Here's how the part is built. I have some questions about the finished solid (model axes, mm). A direction names the side the tool comes from. Round coordinates to 2 decimals unless told otherwise and drop trailing zeros. Loops run counter-clockwise (first coordinate to the right, second up) from the corner with the lowest first, then second, coordinate; pieces in that order, holes last. Notation, with made-up numbers: (-21.75, 40.25) -> (33.25, 40.25) arc R20 ccw to (33.25, 70.25) -> close; hole circle Ø7 at (15, 30.25). An arc over 180 degrees is marked (long way). Use one line per item in the form item = value. Start each with the question number.
Item 1: For faces 4 (the face through (-17, -1.6, -3.3)), 5 (the face through (-0.6, 1.2, 5.9)), 6 (the face through (0, -7.5, 0)), which set-ups out of +Z, -Z, +X, -X, +Y, -Y let a thin tool reach every point of the face, with its end or its side?
Item 2: Thinking about a two-plate mould opening in X: for faces 1 (the face through (-24.16, 6.99, 0.46)), 2 (the face through (-0.4, 0.84, 6.46)), 3 (the face through (0, 7.5, 0)), which applies, released by +X, released by -X, zero draft, split by the parting line, or undercut?
Item 3: If I drill on L1, parallel to X at y = -1.7, z = 1; L2, parallel to X at y = -3.75, z = -3; L3, parallel to Y at x = 20, z = 1.25, over which ranges is the centre line in solid material (lowest first)? Write a range as [from, to].
Item 4: If we section it at B-B (z = 2.75): Write out the boundary of the cut face in (x, y).
Item 5: If we section it at D-D (y = -1.7): State how many separate pieces and enclosed holes the cut face has, then the cut area to 3 significant figures.
Item 6: If we section it at A-A (x = -20): Write out the boundary of the cut face in (y, z), then the cut area to 3 significant figures.
Item 7: If we section it at C-C (x = 13.5): Write out the boundary of the cut face in (y, z).
Item 8: I'm going to push flat-ended pins straight in: pin 1 Ø2 at (x, z) = (-2, 6.5) entering from -Y; pin 2 Ø8 at (x, y) = (20, -1.7) entering from +Z; pin 3 Ø5.5 at (y, z) = (-2, 8) entering from +X. Where does each tip first touch, or does it pass through?
Autodesk Inventor part; units mm, degrees
ref_plane "YZ Plane" through (0, 0, 0) normal (1, 0, 0) x (0, 1, 0)
ref_plane "XZ Plane" through (0, 0, 0) normal (0, 1, 0) x (-1, 0, 0)
ref_plane "XY Plane" through (0, 0, 0) normal (0, 0, 1) x (1, 0, 0)
sketch "Sketch1" plane through (0, 0, 0) normal (0, 0, 1) x (1, 0, 0)
  line L0 (-24.65, 7.5) -> (24.65, 7.5)
  line L1 (24.65, 7.5) -> (24.65, -7.5)
  line L2 (24.65, -7.5) -> (-24.65, -7.5)
  line L3 (-24.65, -7.5) -> (-24.65, 7.5)
  circle A0 centre (-20, -1.7) radius 2
  circle A1 centre (20, -1.7) radius 2
  point P0 (0, 0)
  point P1 (-24.65, 0)
  point P2 (0, 7.5)
  dimension "d0" = 49.3
  dimension "d1" = 15
  dimension "d2" = 4
  dimension "d3" = 40
  dimension "d7" = 9.2
  dimension "d8" = 9.2
  dimension "d9" = 20
extrude "Extrusion1" add sketch "Sketch1" along normal mid plane 9.5
sketch "Sketch2" plane through (0, 0, 4.75) normal (0, 0, 1) x (1, 0, 0)
  line L0 (-6.65, 1.2) -> (5.65, 1.2)
  line L1 (5.65, 1.2) -> (5.65, -4.6)
  line L2 (5.65, -4.6) -> (-6.65, -4.6)
  line L3 (-6.65, -4.6) -> (-6.65, 1.2)
  line L4 (-24.65, 7.5) -> (24.65, 7.5)
  line L5 (24.65, -7.5) -> (24.65, 7.5)
  line L6 (-6.5, 1.2) -> (-6.5, -4.6)
  line L7 (-24.65, -7.5) -> (24.65, -7.5)
  line L8 (5.5, 1.2) -> (5.5, -4.6)
  point P0 (0, 0)
  dimension "d10" = 5.8
  dimension "d11" = 6.3
  dimension "d12" = 12.3
  dimension "d13" = 19
  dimension "d14" = 0.15
extrude "Extrusion3" add sketch "Sketch2" along normal blind 8 contours L0 L8 L2 L6
sketch "Sketch3" plane through (-6.5, 1.2, 4.75) normal (0, 1, 0) x (1, 0, 0)
  line L0 (0, -8) -> (12, -8)
  circle A0 centre (6, -8) radius 6.15
  point P0 (6.5, 4.75)
  dimension "d20" = 12.3
extrude "Extrusion4" cut sketch "Sketch3" against normal blind 8
chamfer "Chamfer1" distance 0.5 angle 45 4 edges at (-6.5, -4.6, 8.075) (-6.5, 1.2, 8.075) (5.5, 1.2, 8.075) (5.5, -4.6, 8.075)
chamfer "Chamfer2" distance 0.5 angle 45 2 edges at (-0.5, -4.6, 6.6) (-0.5, 1.2, 6.6)
fillet "Fillet1" radius 0.2 2 edges at (-6.5, -1.7, 11.4) (5.5, -1.7, 11.4)
chamfer "Chamfer3" distance 1 angle 45 8 edges at (24.65, 0, -4.75) (-24.65, 0, -4.75) (0, 7.5, -4.75) (24.65, 7.5, 0) (-24.65, 7.5, 0) (24.65, -7.5, 0) (0, -7.5, -4.75) (-24.65, -7.5, 0)
sketch "Sketch4" plane through (0, 0, -4.75) normal (0, 0, -1) x (-1, 0, 0)
  circle A0 centre (-20, -1.7) radius 2
  circle A1 centre (-20, -1.7) radius 3
  circle A2 centre (20, -1.7) radius 2
  circle A3 centre (20, -1.7) radius 3
  point P0 (0, 0)
  dimension "d33" = 6
  dimension "d34" = 6
extrude "Extrusion5" cut sketch "Sketch4" against normal blind 3 contours A0 | A1 | A2 | A3
fillet "Fillet2" radius 0.2 8 edges at (0, 7.5, 4.75) (0, -7.5, 4.75) (-24.65, 0, 4.75) (24.65, 0, 4.75) (24.15, 7, 4.75) (24.15, -7, 4.75) (-24.15, -7, 4.75) (-24.15, 7, 4.75)
chamfer "Chamfer4" distance 0.2 angle 45 4 edges at (-22, -1.7, 4.75) (18, -1.7, 4.75) (-22, -1.7, -1.75) (18, -1.7, -1.75)
properties part number "single extruder securer"
Values found:
q1.face_4 = -Z
q1.face_5 = +Z, +X, -X, +Y
q1.face_6 = +Z, -Z, +X, -X, -Y
q2.face_1 = released by -X
q2.face_2 = undercut
q2.face_3 = zero draft
q3.L1 = [-24.65, -22], [-18, 18], [22, 24.65]
q3.L2 = [-24.65, -22.19], [-17.81, 17.81], [22.19, 24.65]
q3.L3 = [-7.5, -3.7], [0.3, 7.5]
q4.outline = (-24.65, -6.5) -> (-23.65, -7.5) -> (23.65, -7.5) -> (24.65, -6.5) -> (24.65, 6.5) -> (23.65, 7.5) -> (-23.65, 7.5) -> (-24.65, 6.5) -> close; hole circle Ø4 at (-20, -1.7); hole circle Ø4 at (20, -1.7)
q5.separate_pieces = 3
q5.enclosed_holes = 0
q5.area = 416 mm2
q6.outline = (-7.5, -3.75) -> (-6.5, -4.75) -> (-4.7, -4.75) -> (-4.7, -1.75) -> (-3.9, -1.75) -> (-3.7, -1.55) -> (-3.7, 4.55) -> (-3.9, 4.75) -> (-7.3, 4.75) arc R0.2 ccw to (-7.5, 4.55) -> close; (0.3, -1.55) -> (0.5, -1.75) -> (1.3, -1.75) -> (1.3, -4.75) -> (6.5, -4.75) -> (7.5, -3.75) -> (7.5, 4.55) arc R0.2 ccw to (7.3, 4.75) -> (0.5, 4.75) -> (0.3, 4.55) -> close
q6.area = 97.4 mm2
q7.outline = (-7.5, -3.75) -> (-6.5, -4.75) -> (6.5, -4.75) -> (7.5, -3.75) -> (7.5, 4.55) arc R0.2 ccw to (7.3, 4.75) -> (-7.3, 4.75) arc R0.2 ccw to (-7.5, 4.55) -> close
q8.pin_1 = -4.6
q8.pin_2 = 4.75
q8.pin_3 = 5.5
